For this review, take the finished solid that the model builds, in its own axes (mm). Face numbers are marked on the shaded views. Coordinates: 2 decimals unless noted, no trailing zeros. Write each loop counter-clockwise with the first axis right and the second up, starting at its lowest first coordinate (ties: lowest second). Pieces come first, ordered by that corner, then holes. Notation, with made-up numbers: (88.5, 37) -> (129.5, 37) arc R16 cw to (129.5, 43) -> close; hole circle Ø6 at (42.25, -31.75). An arc over 180 degrees is marked (long way). One line per item, written item: value. Start each with the question number.
1) For probe 1 along Y at (x, z) = (-3.75, -1.5); probe 2 along X at (y, z) = (3.25, 0.25); probe 3 along Z at (x, y) = (-2.5, 1.75), list the stretches that pass through material, from the lowest coordinate up. Write a range as from..to.
2) Add section B-B (x = 1). State the section outline as (y, z) points, and give its area (3 significant figures).
3) For pin 1 Ø1 at (x, z) = (6, 0) entering from -Y; pin 2 Ø5 at (x, z) = (1, -3) entering from +Y; pin 3 Ø4 at (x, z) = (6, -1) entering from +Y, all flat-tipped, find the tip position at first contact; note any pin that passes through.
4) Add section A-A (x = -3.5). State the section outline as (y, z) points.
5) Mouldability with a two-part tool opening along Z and no side actions: class the marked faces 1, 2, 3 and 4 as released by +Z, released by -Z, zero draft, split by the parting line, or undercut.
Autodesk Inventor part; units mm, degrees
ref_plane "Work Plane1" through (29, 0, 0) normal (0, -1, 0) x (1, 0, 0)
ref_plane "YZ Plane" through (0, 0, 0) normal (1, 0, 0) x (0, 1, 0)
ref_plane "XZ Plane" through (0, 0, 0) normal (0, 1, 0) x (-1, 0, 0)
sketch "Sketch1" plane through (0, 0, 0) normal (0, 0, 1) x (1, 0, 0)
  line L0 (-1.1667, 0) -> (8, 0)
  line L1 (8, 0) -> (8, 2.5)
  line L2 (8, 2.5) -> (2, 2.5)
  line L3 (2, 2.5) -> (1.5091, 2.5)
  line L4 (1.5091, 2.5) -> (0, 2.5)
  line L5 (0, 2.5) -> (0, 4.25)
  line L6 (0, 4.25) -> (-5, 4.25)
  line L7 (-5, 4.25) -> (-5, 2.3094)
  line L8 (-5, 2.3094) -> (-2.5, 2.3094)
  line L9 (-2.5, 2.3094) -> (-1.1667, 0)
  line L10 (-7.6, 0) -> (10.6, 0)
  line L11 (0, -0.85) -> (0, 5.1)
  line L12 (2, 2.5) -> (0, 2.5) construction
  dimension "d1" = 6
  dimension "d2" = 0.4909
  dimension "d3" = 5
  dimension "d4" = 2.5
  dimension "d5" = 60
  dimension "d6" = 5
  dimension "d7" = 5
  dimension "d8" = 4.6188
  dimension "d9" = 8.5
  dimension "d26" = 8
revolve "Body" add sketch "Sketch1" angle 360 about axis through (-1.1667, 0, 0) along (1, 0, 0)
sketch "Sketch2" plane through (-5, 0, 0) normal (-1, 0, 0) x (0, 0, 1)
  circle A0 centre (0, 0) radius 2.3094
  line L0 (0, -5.95) -> (0, 5.95)
  line L1 (-5.95, 0) -> (5.95, 0)
  line L2 (2.3094, 0) -> (1.1547, -2)
  line L3 (1.1547, -2) -> (-1.1547, -2)
  line L4 (-1.1547, -2) -> (-2.3094, 0)
  line L5 (-2.3094, 0) -> (-1.1547, 2)
  line L6 (-1.1547, 2) -> (1.1547, 2)
  line L7 (1.1547, 2) -> (2.3094, 0)
extrude "Slot" add sketch "Sketch2" against normal up to next contours L7 A0 | A0 L2 | L6 L0 A0 | A0 L0 L3 | L0 L6 A0 | A0 L3 L0 | L4 A0 | A0 L5
fillet "Fillet1" radius 0.5 1 edges at (-5, -4.25, 0)
thread "Thread"
chamfer "Chamfer1" distance 0.4908 distance2 0.4908 1 edges at (8, -2.5, 0) measured on face at (8, -0.6238, -0.819)
ref_plane "Work Plane1" through (29, 0, 0) normal (0, -1, 0) x (1, 0, 0)
fillet "Fillet2" radius 0.2 1 edges at (0, -2.5, 0)
equation "\"d1\" = GEL"
equation "\"d3\" = KOH"
equation "\"d4\" = INTI"
equation "\"d6\" = GD"
equation "\"d7\" = BDM"
equation "\"d8\" = 1.1547 * SW"
equation "\"d9\" = KOD"
equation "\"d26\" = NLG"
equation "\"d30\" = R"
equation "\"d17\" = RR"
equation "\"d13\" = GEL"
equation "\"d15\" = -0.5 * SPD + 0.5 * GD"
equation "\"d16\" = GUL"
equation "\"GD\" = NND"
equation "\"NLG\" = 8"
equation "\"GEL\" = 6"
equation "\"KOD\" = 8.5"
equation "\"KOH\" = 5"
equation "\"INTI\" = 2.5"
equation "\"GAL\" = 0.61345 * PTC"
equation "\"GUL\" = 0.61345 * PTC"
equation "\"BDM\" = NND"
equation "\"SW\" = 4"
equation "\"RR\" = 0.5"
equation "\"SPD\" = NND - 1.2269 * PTC"
equation "\"R\" = 0.2"
equation "\"TOA\" = 30deg"
equation "\"GD1\" = THREADDIA - 1.2269 * PTC"
equation "\"THREADDIA\" = 5"
equation "\"FAWI\" = 45deg"
equation "\"ANG\" = 120deg"
equation "\"PTC\" = 0.8"
equation "\"NND\" = 5"
equation "\"E0\" = 1.155 * SW"
properties part number "DIN 912 - M5 x 8" material "Steel, Mild"
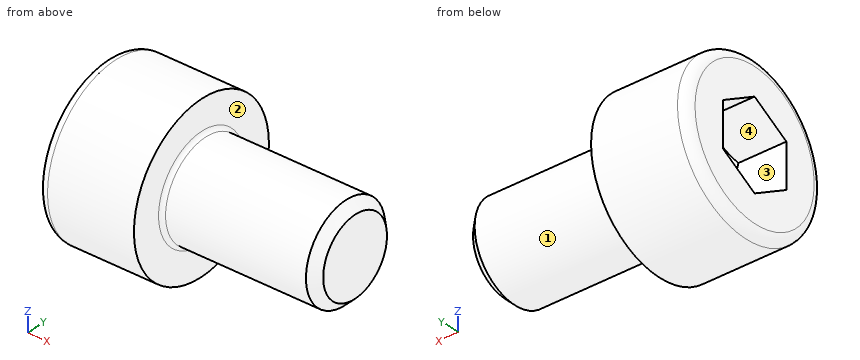
Numbers:
1. probe 1: -3.98..-1.4, 1.4..3.98
1. probe 2: -5..0
1. probe 3: -3.87..-1.3, 1.3..3.87
2. outline: circle Ø5 at (0, 0)
2. area: 19.6 mm²
3. pin 1: y = -2.5
3. pin 2: y = 4.19
3. pin 3: y = 2.5
4. outline: circle Ø8.5 at (0, 0); hole (-2, -1.15) -> (0, -2.31) -> (2, -1.15) -> (2, 1.15) -> (0, 2.31) -> (-2, 1.15) -> close
5. face 1: split by the parting line
5. face 2: zero draft
5. face 3: undercut
5. face 4: undercut
